from build123d import *

# Parameters (mm, degrees)
CUT_EXTRUDE1_START = -10
CUT_EXTRUDE1_DEPTH = 10


with BuildPart() as part:
    # Sketch1 → Revolve1 (revolve)
    with BuildSketch(Plane.XY, mode=Mode.PRIVATE) as revolve1_sk:
        Polygon((0, 65.5), (-2, 65.5), (-2, 54), (-3, 54), (-3, 50), (-12.5, 50), (-12.5, 0), (0, 0), align=None)
    revolve(revolve1_sk.sketch.rotate(Axis((0, 0, 0), (0, 1, 0)), 270), axis=Axis((0, 0, 0), (0, 1, 0)))

    # Sketch2 → Cut-Extrude1 (cut)
    with BuildSketch(Plane(origin=(0, 65.5, 0), x_dir=(1, 0, 0), z_dir=(0, 1, 0)).offset(CUT_EXTRUDE1_START)):
        with BuildLine():
            Line((-1.322875656, 1.5), (-1.322875656, -1.5))
            ThreePointArc((-1.322875656, -1.5), (-2, 0), (-1.322875656, 1.5))
        make_face()
    extrude(amount=CUT_EXTRUDE1_DEPTH, mode=Mode.SUBTRACT)


solid = part.part
Check sheet for the modelled part. Datum: model origin and axes. Units: mm. A direction names the side the tool comes from. Round coordinates to 2 decimals unless told otherwise and drop trailing zeros. Loops run counter-clockwise (first coordinate to the right, second up) from the corner with the lowest first, then second, coordinate; pieces in that order, holes last. Notation, with made-up numbers: (0.25, -28.5) - (5.25, -28.5) arc R7 cw to (5.25, -20.5) - close; hole circle Ø3 at (-39, 78). An arc over 180 degrees is marked (long way). Answer as CSV lines item,"result". Start each with the question number.
Item 1: Section check B-B (x = 0). Record the boundary of the cut face in (y, z), and give its area (3 significant figures).
Item 2: Section check C-C (y = 7.5). Record the boundary of the cut face in (x, z).
Item 3: Scan lines: line 1 (Y direction, x = -7.75, z = 0.5); line 2 (Z direction, x = 1.25, y = 59); line 3 (X direction, y = 44.5, z = -3.75). Record each from-to range of solid material in increasing order. Write a range as [from, to].
Item 4: Set-up check for faces 1 (the flat face through (3, 50, 3)), 2 (the flat face through (0, 0, 0)), 3 (the flat face through (-1.323, 60, 0)): record each of +Z, -Z, +X, -X, +Y, -Y from which the full face is reachable in a straight line by a thin tool's end or side.
Item 5: Section check A-A (z = 0). Record the boundary of the cut face in (x, y).
Item 6: Section check D-D (z = -8.5). Record the boundary of the cut face in (x, y).
Item 7: Depth check by flat-ended pin: P1, Ø2, axis at x = -1.5, y = 45.5, coming from the -Z side; P2, Ø3.5, axis at y = 58, z = 0, coming from the -X side; P3, Ø4, axis at y = 35.5, z = -3, coming from the +X side. Enter the tip coordinate at first touch or a pass-through.
Report:
1,outline,"(0, -12.5) - (50, -12.5) - (50, -3) - (54, -3) - (54, -2) - (65.5, -2) - (65.5, 2) - (54, 2) - (54, 3) - (50, 3) - (50, 12.5) - (0, 12.5) - close"
1,area,"1,320 mm2"
2,outline,"circle Ø25 at (0, 0)"
3,line 1,"y = [0, 50]"
3,line 2,"z = [-1.56, 1.56]"
3,line 3,"x = [-11.92, 11.92]"
4,face 1,"+Y"
4,face 2,"+Z, -Z, +X, -X, -Y"
4,face 3,"+Z, -Z, -X, +Y"
5,outline,"(-12.5, 0) - (12.5, 0) - (12.5, 50) - (3, 50) - (3, 54) - (2, 54) - (2, 65.5) - (-1.32, 65.5) - (-1.32, 55.5) - (-2, 55.5) - (-2, 54) - (-3, 54) - (-3, 50) - (-12.5, 50) - close"
6,outline,"(-9.17, 0) - (9.17, 0) - (9.17, 50) - (-9.17, 50) - close"
7,P1,"stops at z = -12.49"
7,P2,"stops at x = -1.32"
7,P3,"stops at x = 12.46"
